Work out the finished part from the listing and answer in its coordinate system (mm). A direction names the side the tool comes from. Round coordinates to 2 decimals unless told otherwise and drop trailing zeros. Loops run counter-clockwise (first coordinate to the right, second up) from the corner with the lowest first, then second, coordinate; pieces in that order, holes last. Notation, with made-up numbers: M -11,-25 L -5,-25 A21 ccw -5,-15 Z; hole C -27,-12 d5. An arc over 180 degrees is marked long. One line per item, written item: value.
```python
from build123d import *

# Parameters (mm, degrees)
SKETCH1_W                                = 220
SKETCH1_H                                = 217
BLOCO_DEPTH                              = 6
SKETCH2_R                                = 9
SKETCH2_W                                = 28
SKETCH2_H                                = 66
CORTE_MOTOR_DEPTH                        = 155.622928442
RAIOS_5MM_R                              = 5
FUROS_ESCAREADOS_M5_PASSANTE_D           = 5.5
FUROS_ESCAREADOS_M5_PASSANTE_CSINK_D     = 10.4
FUROS_ESCAREADOS_M5_PASSANTE_CSINK_ANGLE = 90


with BuildPart() as part:
    # Sketch1 → Bloco (new body)
    with BuildSketch(Plane(origin=(0, 0, 0), x_dir=(1, 0, 0), z_dir=(0, 1, 0))):
        Rectangle(SKETCH1_W, SKETCH1_H)
    extrude(amount=BLOCO_DEPTH)

    # Sketch2 → Corte Motor (cut, through all)
    with BuildSketch(Plane(origin=(0, 6, 0), x_dir=(1, 0, 0), z_dir=(0, 1, 0))):
        with Locations(Location((0, -8.5, 0), (0, 0, 270))):
            Circle(SKETCH2_R)
        with Locations((96, 63)):
            Rectangle(SKETCH2_W, SKETCH2_H)
    extrude(amount=-CORTE_MOTOR_DEPTH, mode=Mode.SUBTRACT)

    # Raios 5mm
    raios_5mm_edges = [part.edges().sort_by_distance(p)[0] for p in [
        (82, 3, -30),
        (82, 3, -96),
        (110, 3, -30),
    ]]
    fillet(raios_5mm_edges, radius=RAIOS_5MM_R)

    # Furos Escareados - M5 Passante (through all)
    with Locations(Plane(origin=(0, 6, 0), x_dir=(1, 0, 0), z_dir=(0, 1, 0))):
        with Locations((-100, -38.5), (-60, -102.25), (60, -102.25), (100, -38.5), (-60, 102.25), (60, 102.25)):
            CounterSinkHole(FUROS_ESCAREADOS_M5_PASSANTE_D / 2, FUROS_ESCAREADOS_M5_PASSANTE_CSINK_D / 2, counter_sink_angle=FUROS_ESCAREADOS_M5_PASSANTE_CSINK_ANGLE)


solid = part.part
```
1) Each of these flat-tipped pins is pushed along its axis until it touches: pin 1 (9 mm diameter, centred on x = -60, z = 102.25, fed in from +Y); pin 2 (9 mm diameter, centred on x = 100, z = 38.5, fed in from -Y); pin 3 (6.5 mm diameter, centred on x = -100, z = 38.5, fed in from +Y). Where does it stop, or does it pass through?
Check values:
pin 1: y = 5.3
pin 2: y = 0
pin 3: y = 4.05
2) Find section C-C (x = 0). Give the vertices of the cut face in (y, z), then the cut area to 3 significant figures.
Check values:
outline: M 0,-108.5 L 6,-108.5 L 6,-0.5 L 0,-0.5 Z; M 0,17.5 L 6,17.5 L 6,108.5 L 0,108.5 Z
area: 1,190 mm2
3) The mould has two halves that part along Z. Classify faces 1 (the face through (-2, 3, -108.5)), 2 (the face through (-2, 6, -2)), 3 (the face through (82, 3, -63)): +Z half, -Z half, draft (parallel to the pull), parting line (faces both ways), or undercut.
Check values:
face 1: -Z half
face 2: draft
face 3: undercut
4) Find section D-D (y = 1.9). Give the vertices of the cut face in (x, z).
Check values:
outline: M -110,-108.5 L 110,-108.5 L 110,-96 L 87,-96 A5 cw 82,-91 L 82,-35 A5 cw 87,-30 L 105,-30 A5 ccw 110,-25 L 110,108.5 L -110,108.5 Z; hole C -100,38.5 d5.5; hole C -60,-102.25 d5.5; hole C -60,102.25 d5.5; hole C 0,8.5 d18; hole C 60,-102.25 d5.5; hole C 60,102.25 d5.5; hole C 100,38.5 d5.5
5) Find section B-B (z = 8.5). Give the vertices of the cut face in (x, y).
Check values:
outline: M -110,0 L -9,0 L -9,6 L -110,6 Z; M 9,0 L 110,0 L 110,6 L 9,6 Z
6) Find the intervals of material crossed by probe 1 along Z at (x, y) = (-60, 1.2); probe 2 along X at (y, z) = (1.8, 102.25); probe 3 along X at (y, z) = (1.4, 38.5), in increasing order. Write a range as from..to.
Check values:
probe 1: -108.5..-105, -99.5..99.5, 105..108.5
probe 2: -110..-62.75, -57.25..57.25, 62.75..110
probe 3: -110..-102.75, -97.25..97.25, 102.75..110
7) For faces 4 (the face through (-62.65, 3.67, -101.15)), 5 (the face through (96, 3, -30)), determine the directions among +Z, -Z, +X, -X, +Y, -Y from which every point of the face is accessible in a straight line to the end or side of a thin tool.
Check values:
face 4: +Y
face 5: +X, +Y, -Y
8) Find section A-A (x = 60). Give the vertices of the cut face in (y, z).
Check values:
outline: M 0,-108.5 L 6,-108.5 L 6,-107.45 L 3.55,-105 L 0,-105 Z; M 0,-99.5 L 3.55,-99.5 L 6,-97.05 L 6,97.05 L 3.55,99.5 L 0,99.5 Z; M 0,105 L 3.55,105 L 6,107.45 L 6,108.5 L 0,108.5 Z
